Here's the drawing with two shaded views (mm, measured from the low corner). I have some questions. Coordinates: 2 decimals unless noted, no trailing zeros. Order: outer loops, then holes, each group sorted by start corner. A loop starts at its lowest first (then second) coordinate and runs counter-clockwise, first axis right, second up. Notation, with made-up numbers: (-40, 19) -> (-33, 19) arc R26 cw to (-33, 45) -> close; hole circle Ø8 at (-17.75, -17). An arc over 180 degrees is marked (long way). Answer in a Markdown table with one row per item. Add a question column.
1. Imagine slicing it at C-C on y = 6.75. Write out the boundary of the cut face in (x, z).
2. Imagine slicing it at B-B on z = 30. Write out the boundary of the cut face in (x, y), plus the area to 3 significant figures.
3. If I drill on line 1 along X through (y, z) = (3, 53.57); line 2 along Z through (x, y) = (5, 1); line 3 along X through (y, z) = (3, 30), over which ranges is the centre line in solid material (lowest first)? Write a range as [from, to].
4. Will this pin go through, and if not, where does the flat tip stop? pin 1 (1.5 mm diameter, centred on y = 6.5, z = 52, fed in from -X).
5. Imagine slicing it at A-A on z = 6.43. Write out the boundary of the cut face in (x, y).
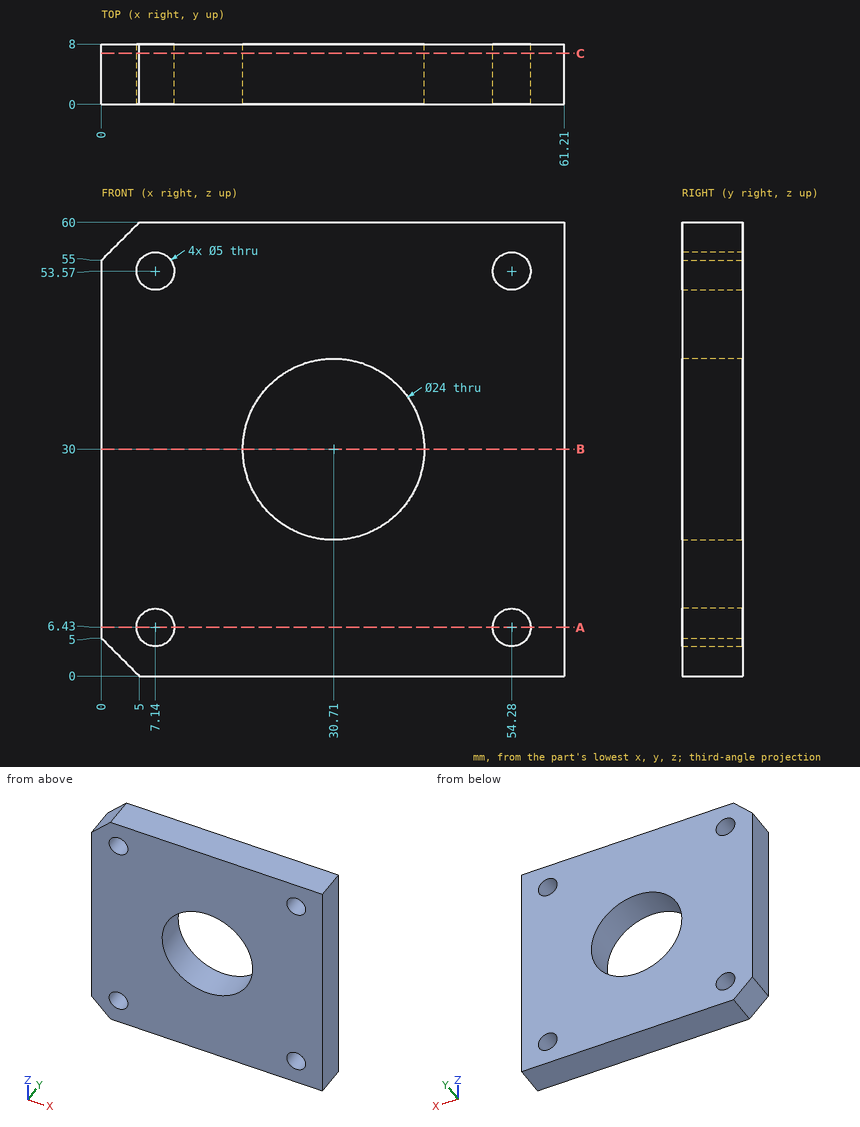
Answers follow:
| question | item | result |
|---|---|---|
| 1 | outline | (0, 5) -> (5, 0) -> (61.21, 0) -> (61.21, 60) -> (5, 60) -> (0, 55) -> close; hole circle Ø5 at (7.14, 6.43); hole circle Ø5 at (7.14, 53.57); hole circle Ø24 at (30.71, 30); hole circle Ø5 at (54.28, 6.43); hole circle Ø5 at (54.28, 53.57) |
| 2 | outline | (0, 0) -> (18.71, 0) -> (18.71, 8) -> (0, 8) -> close; (42.71, 0) -> (61.21, 0) -> (61.21, 8) -> (42.71, 8) -> close |
| 2 | area | 298 mm² |
| 3 | line 1 | x = [0, 4.64], [9.64, 51.78], [56.78, 61.21] |
| 3 | line 2 | z = [0, 5.14], [7.72, 52.28], [54.86, 60] |
| 3 | line 3 | x = [0, 18.71], [42.71, 61.21] |
| 4 | pin 1 | stops at x = 0 |
| 5 | outline | (0, 0) -> (4.64, 0) -> (4.64, 8) -> (0, 8) -> close; (9.64, 0) -> (51.78, 0) -> (51.78, 8) -> (9.64, 8) -> close; (56.78, 0) -> (61.21, 0) -> (61.21, 8) -> (56.78, 8) -> close |
